Build history of the part. All positions in model axes, mm. Face numbers are marked on the shaded views. A direction names the side the tool comes from. Round coordinates to 2 decimals unless told otherwise and drop trailing zeros. Write each loop counter-clockwise with the first axis right and the second up, starting at its lowest first coordinate (ties: lowest second). Pieces come first, ordered by that corner, then holes. Notation, with made-up numbers: (21.5, 43) -> (72.5, 43) arc R29 cw to (72.5, 65) -> close; hole circle Ø7 at (31, 5.5). An arc over 180 degrees is marked (long way). Return JSON: item names as keys, results as strings.
from build123d import *

# Parameters (mm, degrees)
SKETCH1_R           = 92.5
BOSS_EXTRUDE1_DEPTH = 5
SKETCH2_R           = 72
BOSS_EXTRUDE2_DEPTH = 5
SKETCH3_R           = 67
CUT_EXTRUDE1_DEPTH  = 11
SKETCH4_W           = 140
SKETCH4_H           = 70
BOSS_EXTRUDE3_DEPTH = 5
SKETCH6_W           = 60
SKETCH6_H           = 5
BOSS_EXTRUDE4_DEPTH = 20
FILLET1_R           = 2.5
SKETCH7_W           = 110
SKETCH7_H           = 25
BOSS_EXTRUDE5_DEPTH = 5
SKETCH8_W           = 60
SKETCH8_H           = 5
BOSS_EXTRUDE6_DEPTH = 30
SKETCH9_R           = 2
CUT_EXTRUDE2_DEPTH  = 5
SKETCH10_R          = 2
CUT_EXTRUDE3_DEPTH  = 5
SKETCH11_R          = 2
CUT_EXTRUDE4_DEPTH  = 5
SKETCH12_R          = 2.5
CUT_EXTRUDE5_DEPTH  = 5


with BuildPart() as part:
    # Sketch1 → Boss-Extrude1 (new body)
    with BuildSketch(Plane.XY):
        Circle(SKETCH1_R)
    extrude(amount=BOSS_EXTRUDE1_DEPTH)

    # Sketch2 → Boss-Extrude2 (add)
    with BuildSketch(Plane.XY.offset(5)):
        Circle(SKETCH2_R)
    extrude(amount=BOSS_EXTRUDE2_DEPTH)

    # Sketch3 → Cut-Extrude1 (cut, through all)
    with BuildSketch(Plane(origin=(0, 0, 0), x_dir=(-1, 0, 0), z_dir=(0, 0, -1))):
        Circle(SKETCH3_R)
    extrude(amount=-CUT_EXTRUDE1_DEPTH, mode=Mode.SUBTRACT)

    # Sketch4 → Boss-Extrude3 (add)
    with BuildSketch(Plane(origin=(0, 0, 0), x_dir=(-1, 0, 0), z_dir=(0, 0, -1))):
        with Locations((0, -5)):
            Rectangle(SKETCH4_W, SKETCH4_H)
    extrude(amount=-BOSS_EXTRUDE3_DEPTH)

    # Sketch6 → Boss-Extrude4 (add)
    with BuildSketch(Plane.XY.offset(5)):
        with Locations((0, -37.5)):
            Rectangle(SKETCH6_W, SKETCH6_H)
    extrude(amount=BOSS_EXTRUDE4_DEPTH)

    # Fillet1
    fillet1_edges = [part.edges().sort_by_distance(p)[0] for p in [
        (0, -40, 0),
    ]]
    fillet(fillet1_edges, radius=FILLET1_R)

    # Sketch7 → Boss-Extrude5 (add)
    with BuildSketch(Plane(origin=(0, 0, 0), x_dir=(-1, 0, 0), z_dir=(0, 0, -1))):
        with Locations((0, -55)):
            Rectangle(SKETCH7_W, SKETCH7_H)
    extrude(amount=-BOSS_EXTRUDE5_DEPTH)

    # Sketch8 → Boss-Extrude6 (add)
    with BuildSketch(Plane(origin=(0, 0, 0), x_dir=(-1, 0, 0), z_dir=(0, 0, -1))):
        with Locations((0, -45)):
            Rectangle(SKETCH8_W, SKETCH8_H)
    extrude(amount=BOSS_EXTRUDE6_DEPTH)

    # Sketch9 → Cut-Extrude2 (cut)
    with BuildSketch(Plane(origin=(0, -35, 0), x_dir=(1, 0, 0), z_dir=(0, 1, 0))):
        with Locations((-20, -15)):
            Circle(SKETCH9_R)
        with Locations((20, -15)):
            Circle(SKETCH9_R)
    extrude(amount=-CUT_EXTRUDE2_DEPTH, mode=Mode.SUBTRACT)

    # Sketch10 → Cut-Extrude3 (cut)
    with BuildSketch(Plane(origin=(0, -42.5, 0), x_dir=(1, 0, 0), z_dir=(0, 1, 0))):
        with Locations((-20, 20)):
            Circle(SKETCH10_R)
        with Locations((20, 20)):
            Circle(SKETCH10_R)
    extrude(amount=-CUT_EXTRUDE3_DEPTH, mode=Mode.SUBTRACT)

    # Sketch11 → Cut-Extrude4 (cut)
    with BuildSketch(Plane(origin=(0, 0, 0), x_dir=(-1, 0, 0), z_dir=(0, 0, -1))):
        with Locations((-30, -30)):
            Circle(SKETCH11_R)
        with Locations((-30, 20)):
            Circle(SKETCH11_R)
        with Locations((30, 20)):
            Circle(SKETCH11_R)
        with Locations((30, -30)):
            Circle(SKETCH11_R)
    extrude(amount=-CUT_EXTRUDE4_DEPTH, mode=Mode.SUBTRACT)

    # Sketch12 → Cut-Extrude5 (cut)
    with BuildSketch(Plane(origin=(0, 0, 0), x_dir=(-1, 0, 0), z_dir=(0, 0, -1))):
        with Locations((0, -78.5)):
            Circle(SKETCH12_R)
        with Locations((-78.5, 0)):
            Circle(SKETCH12_R)
        with Locations((0, 78.5)):
            Circle(SKETCH12_R)
        with Locations((78.5, 0)):
            Circle(SKETCH12_R)
    extrude(amount=-CUT_EXTRUDE5_DEPTH, mode=Mode.SUBTRACT)


solid = part.part
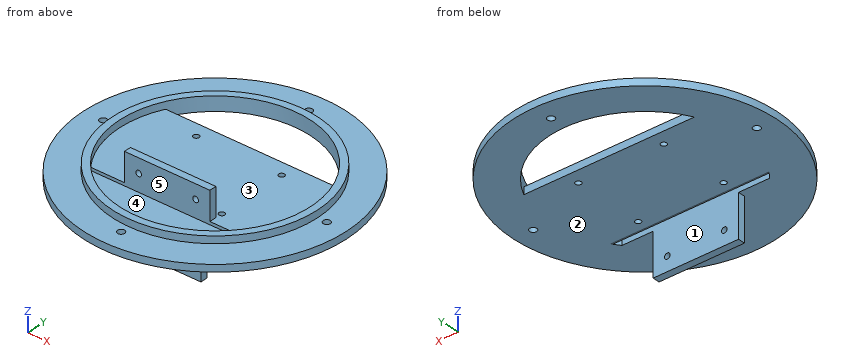
Q1. Saw through at B-B on y = -78.5. List the corners of the cut face in (x, z), then the cut area to 3 significant figures.
Verdict:
{"outline": "(-48.93, 0) -> (-2.5, 0) -> (-2.5, 5) -> (-48.93, 5) -> close; (2.5, 0) -> (48.93, 0) -> (48.93, 5) -> (2.5, 5) -> close", "area": "464 mm²"}
Q2. Pin check, flat tips, straight feed: pin 1 Ø1.5 at (y, z) = (-38.5, 19) entering from +X; pin 2 Ø4.5 at (x, z) = (-20, -20) entering from +Y; pin 3 Ø6 at (x, y) = (15.5, -1) entering from +Z. Stop position of each tip, or through.
Verdict:
{"pin 1": "stops at x = 30", "pin 2": "stops at y = -42.5", "pin 3": "stops at z = 5"}
Q3. Wall check: L1, parallel to X at y = -36.1, z = 15; L2, parallel to Y at x = 0, z = 5.25; L3, parallel to Y at x = 30, z = 3.85. Give the ranges that are in metal, low to high.
Verdict:
{"L1": "x = -30 to -22, -18 to 18, 22 to 30", "L2": "y = -72 to -67, -40 to -35, 67 to 72", "L3": "y = -87.5 to -42.5, -40 to -32, -28 to 18, 22 to 30, 59.91 to 87.5"}
Q4. Saw through at D-D on y = -5.5. List the corners of the cut face in (x, z).
Verdict:
{"outline": "(-92.34, 0) -> (92.34, 0) -> (92.34, 5) -> (71.79, 5) -> (71.79, 10) -> (66.77, 10) -> (66.77, 5) -> (-66.77, 5) -> (-66.77, 10) -> (-71.79, 10) -> (-71.79, 5) -> (-92.34, 5) -> close"}
Q5. 3-axis set-ups, long thin cutter, end or side, ignore diameter. For the marked faces 4 and 5: which of +Z, -Z, +X, -X, +Y, -Y reach the whole face in a straight line?
Verdict:
{"face 4": "+Z", "face 5": "+Z, -Z"}
Q6. Saw through at C-C on x = 43. List the corners of the cut face in (y, z), then the cut area to 3 significant figures.
Verdict:
{"outline": "(-81.9, 0) -> (-42.5, 0) -> (-42.5, 5) -> (-51.38, 5) -> (-51.38, 10) -> (-57.75, 10) -> (-57.75, 5) -> (-81.9, 5) -> close; (-40, 2.5) arc R2.5 ccw to (-37.5, 0) -> (30, 0) -> (30, 5) -> (-40, 5) -> close; (51.38, 0) -> (81.9, 0) -> (81.9, 5) -> (57.75, 5) -> (57.75, 10) -> (51.38, 10) -> close", "area": "762 mm²"}
Q7. Saw through at A-A on x = 0. Count the separate pieces of the cut face and the enclosed holes in it, then the cut area to 3 significant figures.
Verdict:
{"separate pieces": "5", "enclosed holes": "0", "area": "976 mm²"}
Q8. Two-plate mould, pull along Y, no slides. Class the marked faces 1, 2 and 3: +Y half, -Y half, draft (parallel to the pull), parting line (faces both ways), or undercut.
Verdict:
{"face 1": "undercut", "face 2": "draft", "face 3": "undercut"}
